```python
from build123d import *

# Parameters (mm, degrees)
BOSS_EXTRUDE1_DEPTH      = 10
BOSS_EXTRUDE1_DEPTH_BACK = 10
SKETCH1_W                = 40
SKETCH1_H                = 6
BOSS_EXTRUDE2_DEPTH      = 7.5
BOSS_EXTRUDE2_DEPTH_BACK = 7.5
SKETCH1_4_W              = 5
SKETCH1_4_H              = 15
SKETCH2_R                = 2.5
CUT_EXTRUDE1_DEPTH       = 38.960505792
FILLET1_R                = 5


with BuildPart() as part:
    # Sketch1 → Boss-Extrude1 (new, two sides: drawn at the far end of the back side and taken through both)
    with BuildSketch(Plane.XY.offset(-BOSS_EXTRUDE1_DEPTH_BACK)):
        with Locations((20, 3)):
            Rectangle(SKETCH1_W, SKETCH1_H)
    extrude(amount=BOSS_EXTRUDE1_DEPTH + BOSS_EXTRUDE1_DEPTH_BACK)

    # Sketch1_4 → Boss-Extrude2 (add, two sides: drawn at the far end of the back side and taken through both)
    with BuildSketch(Plane.XY.offset(-BOSS_EXTRUDE2_DEPTH_BACK)):
        with Locations((12.5, 13.5)):
            Rectangle(SKETCH1_4_W, SKETCH1_4_H)
        with Locations((27.5, 13.5)):
            Rectangle(SKETCH1_4_W, SKETCH1_4_H)
    extrude(amount=BOSS_EXTRUDE2_DEPTH + BOSS_EXTRUDE2_DEPTH_BACK)

    # Sketch2 → Cut-Extrude1 (cut, through all)
    with BuildSketch(Plane.ZY.offset(-10)):
        with Locations((0, 13.5)):
            Circle(SKETCH2_R)
    extrude(amount=-CUT_EXTRUDE1_DEPTH, mode=Mode.SUBTRACT)

    # Fillet1
    fillet1_edges = [part.edges().sort_by_distance(p)[0] for p in [
        (12.5, 21, 7.5),
        (12.5, 21, -7.5),
        (27.5, 21, 7.5),
        (27.5, 21, -7.5),
    ]]
    fillet(fillet1_edges, radius=FILLET1_R)


solid = part.part
```
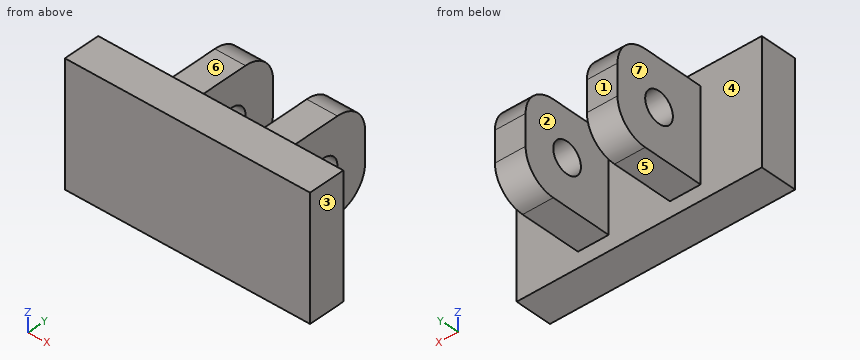
Check sheet for the modelled part. Datum: model origin and axes. Units: mm. Face numbers are marked on the shaded views. A direction names the side the tool comes from. Coordinates: 2 decimals unless noted, no trailing zeros. Loops run counter-clockwise (first coordinate to the right, second up) from the corner with the lowest first, then second, coordinate; pieces in that order, holes last.
1) Sectioned sample at C-C (z = 0). Record the boundary of the cut face in (x, y).
2) Gauge pin test, flat ends, axial feed: pin 1 (12 mm diameter, centred on x = 13.5, z = 6.5, fed in from +Y); pin 2 (7.5 mm diameter, centred on y = 14, z = 2.5, fed in from -X); pin 3 (5.5 mm diameter, centred on x = 27, y = 10.5, fed in from +Z); pin 4 (4 mm diameter, centred on y = 13.5, z = 0, fed in from +X). Record the tip position at first contact, or that the pin passes through.
3) Sectioned sample at B-B (y = 13.5). Record the boundary of the cut face in (x, z).
4) Access from +Z, -Z, +X, -X, +Y, -Y to the whole of each face (thin tool, end or side, straight path). Record for the marked faces 5, 6 and 7.
5) Release check for a two-part mould opening along X. For the marked faces 1, 2, 3 and 4 record: released by +X, released by -X, zero draft, split by the parting line, or undercut.
6) Material ranges on probe 1 along X at (y, z) = (10, 6.5); probe 2 along Y at (x, z) = (11.9, 0); probe 3 along Y at (x, z) = (17, 2.25), recorded low to high.
7) Sectioned sample at A-A (x = 11.5). Record the boundary of the cut face in (y, z), and give its area (3 significant figures).
8) Sectioned sample at D-D (z = 6.5). Record the boundary of the cut face in (x, y), and give its area (3 significant figures).
Check sheet entries:
1. outline: (0, 0) - (40, 0) - (40, 6) - (30, 6) - (30, 11) - (25, 11) - (25, 6) - (15, 6) - (15, 11) - (10, 11) - (10, 6) - (0, 6) - close; (10, 16) - (15, 16) - (15, 21) - (10, 21) - close; (25, 16) - (30, 16) - (30, 21) - (25, 21) - close
2. pin 1: stops at y = 21
2. pin 2: stops at x = 10
2. pin 3: stops at z = 7.5
2. pin 4: passes through
3. outline: (10, -7.5) - (15, -7.5) - (15, -2.5) - (10, -2.5) - close; (10, 2.5) - (15, 2.5) - (15, 7.5) - (10, 7.5) - close; (25, -7.5) - (30, -7.5) - (30, -2.5) - (25, -2.5) - close; (25, 2.5) - (30, 2.5) - (30, 7.5) - (25, 7.5) - close
4. face 5: -Z, +X, -X, +Y
4. face 6: +Z, +X, -X, +Y
4. face 7: +Z, -Z, -X, +Y
5. face 1: zero draft
5. face 2: undercut
5. face 3: released by +X
5. face 4: undercut
6. probe 1: x = 10 to 15, 25 to 30
6. probe 2: y = 0 to 11, 16 to 21
6. probe 3: y = 0 to 6
7. outline: (0, -10) - (6, -10) - (6, -7.5) - (16, -7.5) arc R5 ccw to (21, -2.5) - (21, 2.5) arc R5 ccw to (16, 7.5) - (6, 7.5) - (6, 10) - (0, 10) - close; hole circle Ø5 at (13.5, 0)
7. area: 315 mm2
8. outline: (0, 0) - (40, 0) - (40, 6) - (30, 6) - (30, 19) - (25, 19) - (25, 6) - (15, 6) - (15, 19) - (10, 19) - (10, 6) - (0, 6) - close
8. area: 370 mm2
